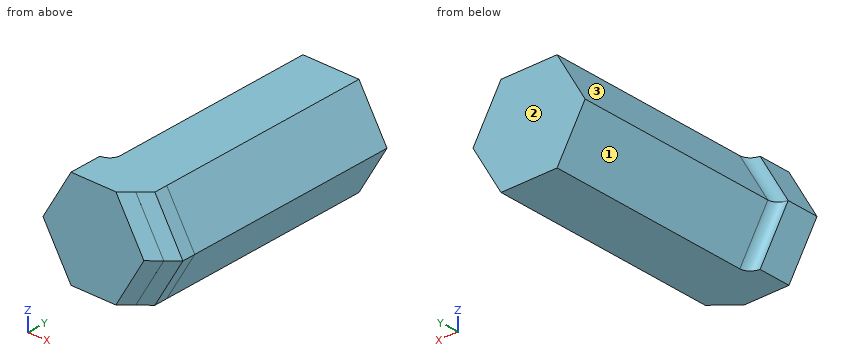
from build123d import *

# Parameters (mm, degrees)
EXTRUDE_1_DEPTH = 20
EXTRUDE_2_DEPTH = 3
CHAMFER_1_SIZE  = 2.1
CHAMFER_2_SIZE  = 0.9
FILLET_2_R      = 1


# Some blends are built 0.0001 mm under size
with BuildPart() as part:
    # 草图1 → 凸台-拉伸1 (new body)
    with BuildSketch(Plane(origin=(0, 0, 0), x_dir=(1, 0, 0), z_dir=(0, 1, 0))):
        Polygon((2.598076211, -4.5), (5.196152423, 0), (2.598076211, 4.5), (-2.598076211, 4.5), (-5.196152423, 0), (-2.598076211, -4.5), align=None)
    extrude(amount=EXTRUDE_1_DEPTH)

    # 草图2 → 凸台-拉伸2 (add)
    with BuildSketch(Plane(origin=(0, 0, 0), x_dir=(-1, 0, 0), z_dir=(0, -1, 0))):
        Polygon((6.196152423, 0), (3.598076211, 4.5), (-1.598076211, 4.5), (-4.196152423, 0), (-1.598076211, -4.5), (3.598076211, -4.5), align=None)
    extrude(amount=EXTRUDE_2_DEPTH)

    # 倒角1
    # the kernel refuses this chamfer: 2.1 mm, written as the material it adds along each edge
    with BuildSketch(Plane(origin=(-1.102190926, 0, -9.176999876), x_dir=(0.8656979742248804, 0.027495876610586372, -0.49981095845564816), z_dir=(0.49999999999999983, 0, 0.8660254037844388))) as chamfer_1_piece_1_section:
        Polygon((CHAMFER_1_SIZE * 0.999621916911, -CHAMFER_1_SIZE * 0.0274958766106), (-CHAMFER_1_SIZE * 0.0274958766106, -CHAMFER_1_SIZE * 0.999621916911), (0, 0), align=None)
    chamfer_1_piece_1 = extrude(amount=15.997220972, mode=Mode.PRIVATE)
    chamfer_1_piece_1 = split(chamfer_1_piece_1, bisect_by=Plane(origin=(3.647114317, -0.87342855, -2.683012702), z_dir=(-0.8660254037844421, 0, 0.49999999999999406)), keep=Keep.TOP, mode=Mode.PRIVATE)
    chamfer_1_piece_1 = split(chamfer_1_piece_1, bisect_by=Plane(origin=(3.19992905, -0.87342855, -4.5), z_dir=(0, 0, 1)), keep=Keep.TOP, mode=Mode.PRIVATE)
    chamfer_1_piece_1 = split(chamfer_1_piece_1, bisect_by=Plane(origin=(4.997078842, -0.87342855, -1.387245251), z_dir=(-0.8660254037844387, 0, -0.5000000000000003)), keep=Keep.TOP, mode=Mode.PRIVATE)
    add(chamfer_1_piece_1)
    with BuildSketch(Plane(origin=(6.89641956, 0, -4.676999876), x_dir=(0.8656979742248802, 0.027495876610586358, 0.49981095845564866), z_dir=(-0.5000000000000003, 0, 0.8660254037844386))) as chamfer_1_piece_2_section:
        Polygon((CHAMFER_1_SIZE * 0.999621916911, -CHAMFER_1_SIZE * 0.0274958766106), (-CHAMFER_1_SIZE * 0.0274958766106, -CHAMFER_1_SIZE * 0.999621916911), (0, 0), align=None)
    chamfer_1_piece_2 = extrude(amount=15.997220972, mode=Mode.PRIVATE)
    chamfer_1_piece_2 = split(chamfer_1_piece_2, bisect_by=Plane(origin=(3.647114317, -0.87342855, 2.683012702), z_dir=(-0.8660254037844353, 0, -0.500000000000006)), keep=Keep.TOP, mode=Mode.PRIVATE)
    chamfer_1_piece_2 = split(chamfer_1_piece_2, bisect_by=Plane(origin=(3.19992905, -0.87342855, 4.5), z_dir=(0, 0, -1)), keep=Keep.TOP, mode=Mode.PRIVATE)
    chamfer_1_piece_2 = split(chamfer_1_piece_2, bisect_by=Plane(origin=(4.997078842, -0.87342855, 1.387245251), z_dir=(-0.8660254037844388, 0, 0.49999999999999983)), keep=Keep.TOP, mode=Mode.PRIVATE)
    add(chamfer_1_piece_2)
    with BuildSketch(Plane(origin=(6.89641956, 0, -4.676999876), x_dir=(0.8656979742248802, 0.027495876610586358, 0.49981095845564866), z_dir=(-0.5000000000000003, 0, 0.8660254037844386))) as chamfer_1_piece_3a_section:
        Polygon((CHAMFER_1_SIZE * 0.999621916911, -CHAMFER_1_SIZE * 0.0274958766106), (-CHAMFER_1_SIZE * 0.0274958766106, -CHAMFER_1_SIZE * 0.999621916911), (0, 0), align=None)
    chamfer_1_piece_3a = extrude(amount=15.997220972, mode=Mode.PRIVATE)
    chamfer_1_piece_3a = split(chamfer_1_piece_3a, bisect_by=Plane(origin=(5.090413844, -0.863604647, 0.183144591), z_dir=(-0.8660254037844353, 0, -0.500000000000006)), keep=Keep.TOP, mode=Mode.PRIVATE)
    chamfer_1_piece_3a = split(chamfer_1_piece_3a, bisect_by=Plane(origin=(5.032629581, -0.863604647, -0.28322987), z_dir=(-0.8660254037844421, 0, 0.49999999999999406)), keep=Keep.TOP, mode=Mode.PRIVATE)
    chamfer_1_piece_3a = split(chamfer_1_piece_3a, bisect_by=Plane(origin=(4.282629581, -0.863604647, 0.149782832), z_dir=(0.8660254037844388, 0, -0.49999999999999983)), keep=Keep.TOP, mode=Mode.PRIVATE)
    with BuildSketch(Plane(origin=(-1.102190926, 0, -9.176999876), x_dir=(0.8656979742248804, 0.027495876610586372, -0.49981095845564816), z_dir=(0.49999999999999983, 0, 0.8660254037844388))) as chamfer_1_piece_3b_section:
        Polygon((CHAMFER_1_SIZE * 0.999621916911, -CHAMFER_1_SIZE * 0.0274958766106), (-CHAMFER_1_SIZE * 0.0274958766106, -CHAMFER_1_SIZE * 0.999621916911), (0, 0), align=None)
    chamfer_1_piece_3b = extrude(amount=15.997220972, mode=Mode.PRIVATE)
    chamfer_1_piece_3b = split(chamfer_1_piece_3b, bisect_by=Plane(origin=(5.032629581, -0.863604647, 0.28322987), z_dir=(-0.8660254037844353, 0, -0.500000000000006)), keep=Keep.TOP, mode=Mode.PRIVATE)
    chamfer_1_piece_3b = split(chamfer_1_piece_3b, bisect_by=Plane(origin=(5.090413844, -0.863604647, -0.183144591), z_dir=(-0.8660254037844421, 0, 0.49999999999999406)), keep=Keep.TOP, mode=Mode.PRIVATE)
    chamfer_1_piece_3b = split(chamfer_1_piece_3b, bisect_by=Plane(origin=(4.282629581, -0.863604647, -0.149782832), z_dir=(0.8660254037844387, 0, 0.5000000000000003)), keep=Keep.TOP, mode=Mode.PRIVATE)
    chamfer_1_piece_3 = chamfer_1_piece_3a & chamfer_1_piece_3b
    add(chamfer_1_piece_3)

    # 倒角2
    chamfer_2_edges = [part.edges().sort_by_distance(p)[0] for p in [
        (2.897114317, -3, 2.25),
        (2.897114317, -3, -2.25),
    ]]
    chamfer(chamfer_2_edges, length=CHAMFER_2_SIZE - 0.0001)  # a hair under: the kernel refuses the full size

    # 圆角2
    # the kernel refuses this fillet: 1 mm, written as the material it adds along each edge
    with BuildSketch(Plane(origin=(-1.359345253, 0, -6.645544957), x_dir=(-0.8660254037844353, 5.384295521873835e-15, -0.500000000000006), z_dir=(-0.500000000000006, 0, 0.8660254037844353))) as fillet_2_piece_1_section:
        with BuildLine():
            CenterArc((1, -0.990984767), FILLET_2_R, 97.699329946, 82.300670054)
            Line((0, -0.990984767), (-0.02, -0.990984767))
            Line((-0.02, -0.990984767), (-0.02, 0))
            Line((-0.02, 0), (0, 0.02))
            ThreePointArc((0, 0.02), (0.433012702, 0.02), (0.863345912, 0.019819695))
            Line((0.863345912, 0.019819695), (0.866025404, 0))
        make_face()
    fillet_2_piece_1 = extrude(amount=10.151076256, mode=Mode.PRIVATE)
    fillet_2_piece_1 = split(fillet_2_piece_1, bisect_by=Plane(origin=(-4.072160792, 0.234330223, -4.5), z_dir=(0, 0, 1)), keep=Keep.TOP, mode=Mode.PRIVATE)
    fillet_2_piece_1 = split(fillet_2_piece_1, bisect_by=Plane(origin=(-5.933194713, 0.234330223, -1.276594694), z_dir=(0.8660254037844423, 0, -0.49999999999999395)), keep=Keep.TOP, mode=Mode.PRIVATE)
    add(fillet_2_piece_1)
    with BuildSketch(Plane(origin=(-6.434883381, 0, -2.145544957), x_dir=(-0.8660254037844421, 5.3842955218737e-15, 0.4999999999999939), z_dir=(0.49999999999999395, 0, 0.8660254037844423))) as fillet_2_piece_2_section:
        with BuildLine():
            CenterArc((1, -0.990984767), FILLET_2_R, 97.699329946, 82.300670054)
            Line((0, -0.990984767), (-0.02, -0.990984767))
            Line((-0.02, -0.990984767), (-0.02, 0))
            Line((-0.02, 0), (0, 0.02))
            ThreePointArc((0, 0.02), (0.433012702, 0.02), (0.863345912, 0.019819695))
            Line((0.863345912, 0.019819695), (0.866025404, 0))
        make_face()
    fillet_2_piece_2 = extrude(amount=10.151076256, mode=Mode.PRIVATE)
    fillet_2_piece_2 = split(fillet_2_piece_2, bisect_by=Plane(origin=(-4.072160792, 0.234330223, 4.5), z_dir=(0, 0, -1)), keep=Keep.TOP, mode=Mode.PRIVATE)
    fillet_2_piece_2 = split(fillet_2_piece_2, bisect_by=Plane(origin=(-5.933194713, 0.234330223, 1.276594694), z_dir=(0.8660254037844353, 0, 0.500000000000006)), keep=Keep.TOP, mode=Mode.PRIVATE)
    add(fillet_2_piece_2)
    with BuildSketch(Plane(origin=(-6.434883381, 0, -2.145544957), x_dir=(-0.8660254037844421, 5.3842955218737e-15, 0.4999999999999939), z_dir=(0.49999999999999395, 0, 0.8660254037844423))) as fillet_2_piece_3a_section:
        with BuildLine():
            CenterArc((1, -0.990984767), FILLET_2_R, 97.699329946, 82.300670054)
            Line((0, -0.990984767), (-0.02, -0.990984767))
            Line((-0.02, -0.990984767), (-0.02, 0))
            Line((-0.02, 0), (0, 0.02))
            ThreePointArc((0, 0.02), (0.433012702, 0.02), (0.863345912, 0.019819695))
            Line((0.863345912, 0.019819695), (0.866025404, 0))
        make_face()
    fillet_2_piece_3a = extrude(amount=10.151076256, mode=Mode.PRIVATE)
    fillet_2_piece_3a = split(fillet_2_piece_3a, bisect_by=Plane(origin=(-5.943047398, 0.228517216, -0.438390763), z_dir=(0.8660254037844385, 0, 0.5000000000000004)), keep=Keep.TOP, mode=Mode.PRIVATE)
    fillet_2_piece_3a = split(fillet_2_piece_3a, bisect_by=Plane(origin=(-5.193047398, 0.228517216, -0.005378061), z_dir=(-0.8660254037844353, 0, -0.500000000000006)), keep=Keep.TOP, mode=Mode.PRIVATE)
    with BuildSketch(Plane(origin=(-1.359345253, 0, -6.645544957), x_dir=(-0.8660254037844353, 5.384295521873835e-15, -0.500000000000006), z_dir=(-0.500000000000006, 0, 0.8660254037844353))) as fillet_2_piece_3b_section:
        with BuildLine():
            CenterArc((1, -0.990984767), FILLET_2_R, 97.699329946, 82.300670054)
            Line((0, -0.990984767), (-0.02, -0.990984767))
            Line((-0.02, -0.990984767), (-0.02, 0))
            Line((-0.02, 0), (0, 0.02))
            ThreePointArc((0, 0.02), (0.433012702, 0.02), (0.863345912, 0.019819695))
            Line((0.863345912, 0.019819695), (0.866025404, 0))
        make_face()
    fillet_2_piece_3b = extrude(amount=10.151076256, mode=Mode.PRIVATE)
    fillet_2_piece_3b = split(fillet_2_piece_3b, bisect_by=Plane(origin=(-5.943047398, 0.228517216, 0.438390763), z_dir=(0.8660254037844388, 0, -0.49999999999999967)), keep=Keep.TOP, mode=Mode.PRIVATE)
    fillet_2_piece_3b = split(fillet_2_piece_3b, bisect_by=Plane(origin=(-5.193047398, 0.228517216, 0.005378061), z_dir=(-0.8660254037844423, 0, 0.49999999999999395)), keep=Keep.TOP, mode=Mode.PRIVATE)
    fillet_2_piece_3 = fillet_2_piece_3a & fillet_2_piece_3b
    add(fillet_2_piece_3)


solid = part.part
Model file for the job. Use its own axes, mm. Face numbers are marked on the shaded views. A direction names the side the tool comes from. Give positions to 0.01 mm unless a question says otherwise; leave off trailing zeros. Order: outer loops, then holes, each group sorted by start corner. A loop starts at its lowest first (then second) coordinate and runs counter-clockwise, first axis right, second up. Notation, with made-up numbers: (67, 23.5) - (98, 23.5) arc R13 cw to (98, 42.5) - close; hole circle Ø7 at (13, 89.5). An arc over 180 degrees is marked (long way). Write item = value, one per line. Start each with the question number.
1. Which spindle directions (+Z, -Z, +X, -X, +Y, -Y) get a long thin tool onto all of the face, cutting with end or side? Do the marked faces 1, 2 and 3. Say none if no direction does.
2. Probe line 1 along X through (y, z) = (16.5, 2.75); line 2 along X through (y, z) = (3, 3.25); line 3 along Z through (x, y) = (4, 11.75). List the from-to ranges inside material, lowest first.
3. Cut at C-C, the plane y = -0.25. List the corners of the cut face in (x, z), and give its area (3 significant figures).
4. Cut at A-A, the plane y = 14.5. List the corners of the cut face in (x, z).
Taken from the geometry:
q1.face_1 = -Z, -X, +Y
q1.face_2 = +Z, -Z, +X, -X, +Y
q1.face_3 = +Z, -X, +Y
q2.line_1 = -3.61 to 3.61
q2.line_2 = -3.32 to 3.32
q2.line_3 = -2.07 to 2.07
q3.outline = (-6.2, 0) - (-3.6, -4.5) - (2.6, -4.5) - (5.2, 0) - (2.6, 4.5) - (-3.6, 4.5) - close
q3.area = 79.1 mm²
q4.outline = (-5.2, 0) - (-2.6, -4.5) - (2.6, -4.5) - (5.2, 0) - (2.6, 4.5) - (-2.6, 4.5) - close
